The listing builds one solid part. Answer for the finished solid, in the listing's coordinates (mm). A direction names the side the tool comes from. Round coordinates to 2 decimals unless told otherwise and drop trailing zeros. Write each loop counter-clockwise with the first axis right and the second up, starting at its lowest first coordinate (ties: lowest second). Pieces come first, ordered by that corner, then holes.
Autodesk Inventor part; units mm, degrees
ref_plane "YZ Plane" through (0, 0, 0) normal (1, 0, 0) x (0, 1, 0)
ref_plane "XZ Plane" through (0, 0, 0) normal (0, 1, 0) x (-1, 0, 0)
ref_plane "XY Plane" through (0, 0, 0) normal (0, 0, 1) x (1, 0, 0)
sketch "Skizze1" plane through (0, 0, 0) normal (0, 0, 1) x (1, 0, 0)
  line L0 (-22.5, -25) -> (22.5, -25)
  line L1 (22.5, -25) -> (22.5, 25)
  line L2 (22.5, 25) -> (-22.5, 25)
  line L3 (-22.5, 25) -> (-22.5, -25)
  line L4 (-22.5, -25) -> (22.5, 25) construction
  line L5 (22.5, -25) -> (-22.5, 25) construction
  line L6 (0, 11) -> (0, -11) construction
  line L7 (-15.25, 18.75) -> (15.25, 18.75) construction
  line L8 (15.25, 18.75) -> (15.25, 3.25) construction
  line L9 (15.25, 3.25) -> (-15.25, 3.25) construction
  line L10 (-15.25, 3.25) -> (-15.25, 18.75) construction
  line L11 (-15.25, 18.75) -> (15.25, 3.25) construction
  line L12 (15.25, 18.75) -> (-15.25, 3.25) construction
  line L13 (-17.7097, 20) -> (17.7097, 20) construction
  line L14 (17.7097, 20) -> (17.7097, 2) construction
  line L15 (17.7097, 2) -> (-17.7097, 2) construction
  line L16 (-17.7097, 2) -> (-17.7097, 20) construction
  line L17 (-17.7097, 20) -> (17.7097, 2) construction
  line L18 (17.7097, 20) -> (-17.7097, 2) construction
  line L19 (-15.25, -18.75) -> (15.25, -18.75) construction
  line L20 (15.25, -18.75) -> (15.25, -3.25) construction
  line L21 (15.25, -3.25) -> (-15.25, -3.25) construction
  line L22 (-15.25, -3.25) -> (-15.25, -18.75) construction
  line L23 (-15.25, -18.75) -> (15.25, -3.25) construction
  line L24 (15.25, -18.75) -> (-15.25, -3.25) construction
  circle A0 centre (-15.25, 18.75) radius 1.25
  circle A1 centre (15.25, 3.25) radius 1.25
  circle A2 centre (15.25, -18.75) radius 1.25
  circle A3 centre (-15.25, -3.25) radius 1.25
  point P0 (0, 0)
  point P1 (0, 0)
  dimension "d0" = 45
  dimension "d1" = 15.5
  dimension "d2" = 30.5
  dimension "d3" = 2
  dimension "d4" = 18
  dimension "d5" = 25
  dimension "d6" = 2.5
extrude "Extrusion1" add sketch "Skizze1" along normal blind 3
fillet "Rundung1" radius 6 4 edges at (-22.5, 25, 1.5) (-22.5, -25, 1.5) (22.5, -25, 1.5) (22.5, 25, 1.5)
chamfer "Fase1" distance 2 angle 45 4 edges at (-16.5, -3.25, 0) (14, -18.75, 0) (14, 3.25, 0) (-16.5, 18.75, 0)
sketch "Skizze2" plane through (0, 0, 3) normal (0, 0, 1) x (1, 0, 0)
  arc A0 (22.5, 19) -> (16.5, 25) centre (16.5, 19) ccw
  line L0 (16.5, 25) -> (-16.5, 25)
  arc A1 (-16.5, 25) -> (-22.5, 19) centre (-16.5, 19) ccw
  line L1 (-22.5, 19) -> (-22.5, -19)
  arc A2 (-22.5, -19) -> (-16.5, -25) centre (-16.5, -19) ccw
  line L2 (-16.5, -25) -> (16.5, -25)
  arc A3 (16.5, -25) -> (22.5, -19) centre (16.5, -19) ccw
  line L3 (22.5, -19) -> (22.5, 19)
  circle A4 centre (-15.25, -3.25) radius 1.25
  circle A5 centre (15.25, -18.75) radius 1.25
  circle A6 centre (15.25, 3.25) radius 1.25
  circle A7 centre (-15.25, 18.75) radius 1.25
  circle A8 centre (15.25, 3.25) radius 4
  circle A9 centre (15.25, -18.75) radius 4
  circle A10 centre (-15.25, -3.25) radius 4
  circle A11 centre (-15.25, 18.75) radius 4
  line L4 (15.25, -18.75) -> (15.25, 18.75) construction
  line L5 (19.25, -18.75) -> (19.25, 18.75)
  line L6 (11.25, 18.75) -> (11.25, -18.75)
  arc A12 (11.25, -18.75) -> (19.25, -18.75) centre (15.25, -18.75) ccw
  arc A13 (19.25, 18.75) -> (11.25, 18.75) centre (15.25, 18.75) ccw
  line L7 (-15.25, 18.75) -> (-15.25, -18.75) construction
  line L8 (-19.25, 18.75) -> (-19.25, -18.75)
  line L9 (-11.25, -18.75) -> (-11.25, 18.75)
  arc A14 (-11.25, 18.75) -> (-19.25, 18.75) centre (-15.25, 18.75) ccw
  arc A15 (-19.25, -18.75) -> (-11.25, -18.75) centre (-15.25, -18.75) ccw
  line L10 (-15.25, -18.75) -> (15.25, -18.75) construction
  line L11 (15.25, 18.75) -> (-15.25, 18.75) construction
  point P0 (0, 0)
  point P1 (15.25, 0)
  point P2 (-15.25, 0)
  dimension "d13" = 8
extrude "Extrusion2" add sketch "Skizze2" along normal blind 2 contours A8 | L5 A9 L6 A8 | A8 L6 A13 L5 | A9 | A10 | L9 A15 L8 A10 | A10 L8 A11 L9 | A11
chamfer "Fase3" distance 2 angle 45 8 edges at (15.25, 22.75, 3) (19.25, 0, 3) (15.25, -22.75, 3) (11.25, 0, 3) (-15.25, 22.75, 3) (-11.25, 0, 3) (-15.25, -22.75, 3) (-19.25, 0, 3)
sketch "Skizze4" plane through (0, 0, 3) normal (0, 0, 1) x (1, 0, 0)
  line L0 (-6, 20) -> (6, 20) construction
  line L1 (-6, 21.5) -> (6, 21.5)
  line L2 (6, 18.5) -> (-6, 18.5)
  arc A0 (-6, 21.5) -> (-6, 18.5) centre (-6, 20) ccw
  arc A1 (6, 18.5) -> (6, 21.5) centre (6, 20) ccw
  line L3 (-6, -20) -> (6, -20) construction
  line L4 (-6, -18.5) -> (6, -18.5)
  line L5 (6, -21.5) -> (-6, -21.5)
  arc A2 (-6, -18.5) -> (-6, -21.5) centre (-6, -20) ccw
  arc A3 (6, -21.5) -> (6, -18.5) centre (6, -20) ccw
  line L6 (0, -20) -> (0, 20)
  point P0 (0, 0)
  point P1 (0, 0)
  dimension "d22" = 3
  dimension "d23" = 12
  dimension "d24" = 40
extrude "Extrusion3" cut sketch "Skizze4" against normal through all
chamfer "Fase4" distance 1 angle 45 8 edges at (7.5, 20, 3) (0, 18.5, 3) (-7.5, 20, 3) (0, 21.5, 3) (7.5, -20, 3) (0, -21.5, 3) (-7.5, -20, 3) (0, -18.5, 3)
properties part number "wandler"
1. A tool of negligible diameter and unlimited length cuts with its end or side. For faces 1 (the face through (14.952, -17.408, 1.875)), 2 (the face through (7.7, -20, 2.2)), 3 (the face through (0, -21.5, 1)), from which of +Z, -Z, +X, -X, +Y, -Y can it reach the whole face along a straight path? Write none if from no direction.
Geometry says:
face 1: -Z
face 2: +Z
face 3: +Z, -Z
2. Given pin 1 (1.5 mm diameter, centred on x = 17.5, z = 2.5, fed in from +Y); pin 2 (4 mm diameter, centred on x = -15.5, y = -4, fed in from -Z); pin 3 (2 mm diameter, centred on x = -15.25, y = 18.75, fed in from +Z), each flat-ended and moving along its own axis, determine where each tip first touches the part or whether it passes through.
Geometry says:
pin 1: stops at y = 24.99
pin 2: stops at z = 0.46
pin 3: passes through
3. Straight lines are drawn through the part: line 1 along Y through (x, z) = (1, 0.75); line 2 along Y through (x, z) = (-15.25, 4); line 3 along Z through (x, y) = (-7, 17.5). For each, find the intervals that lie inside material, in ascending order.
Geometry says:
line 1: y = -25 to -21.5, -18.5 to 18.5, 21.5 to 25
line 2: y = -23.75 to -4.5, -2 to 17.5, 20 to 23.75
line 3: z = 0 to 3
4. Section C-C on z = 0.8 is taken. Determine the outline of the cut face in (x, y), plus the area to 3 significant figures.
Geometry says:
outline: (-22.5, -19) arc R6 ccw to (-16.5, -25) - (16.5, -25) arc R6 ccw to (22.5, -19) - (22.5, 19) arc R6 ccw to (16.5, 25) - (-16.5, 25) arc R6 ccw to (-22.5, 19) - close; hole circle Ø4.9 at (-15.25, -3.25); hole circle Ø4.9 at (-15.25, 18.75); hole (-6, -21.5) - (6, -21.5) arc R1.5 ccw to (6, -18.5) - (-6, -18.5) arc R1.5 ccw to start; hole (-6, 18.5) - (6, 18.5) arc R1.5 ccw to (6, 21.5) - (-6, 21.5) arc R1.5 ccw to start; hole circle Ø4.9 at (15.25, -18.75); hole circle Ø4.9 at (15.25, 3.25)
area: 2,060 mm2
5. For a pull along X with two mould halves and no side action, classify faces 4 (the face through (-20.696, 23.289, 1.521)), 5 (the face through (-7.5, -20, 1)), 6 (the face through (0, -25, 1)) as released by +X, released by -X, zero draft, split by the parting line, or undercut.
Geometry says:
face 4: released by -X
face 5: undercut
face 6: zero draft
6. Section A-A on x = 15.25 is taken. Give the number of separate pieces and of enclosed holes in the cut face, plus the area to 3 significant figures.
Geometry says:
separate pieces: 3
enclosed holes: 0
area: 212 mm2
